Read the model definition and answer for the solid it produces. Units are mm, in the model's axes. A direction names the side the tool comes from. Give positions to 0.01 mm unless a question says otherwise; leave off trailing zeros. Loops run counter-clockwise (first coordinate to the right, second up) from the corner with the lowest first, then second, coordinate; pieces in that order, holes last. Notation, with made-up numbers: M 84,7.5 L 134,7.5 A28 cw 134,44.5 Z; hole C 69,86 d6. An arc over 180 degrees is marked long. Return JSON: item names as keys, results as strings. Group by question number.
```python
from build123d import *

# Parameters (mm, degrees)
F0_R     = 17.5
F1_DEPTH = 75
F4_R     = 15
F5_DEPTH = 25


with BuildPart() as f1:
    # F0 (on Top) → F1 (new body)
    with BuildSketch(Plane.XY):
        Circle(F0_R)
    extrude(amount=F1_DEPTH)

    # F2 (on Front) → F3 (revolve)
    with BuildSketch(Plane.XZ):
        Polygon((-19.5, 74), (0, 74), (0, 123), (-16.75, 123), (-23.75, 116), (-23.75, 104), (-19.5, 99.75), align=None)
    revolve(axis=Axis((0, 0, 40.698601), (0, 0, 1)))

    # F4 (on face) → F5 (join)
    with BuildSketch(Plane.XY.offset(123)):
        Circle(F4_R)
    extrude(amount=F5_DEPTH)


solid = f1.part
```
1. Straight lines are drawn through the part: line 1 along Z through (x, y) = (-3.5, 16); line 2 along Y through (x, z) = (0.5, 142); line 3 along Y through (x, z) = (0, 47). For each, find the intervals that lie inside material, in ascending order.
2. Flat-ended cylindrical pins translate along their axes: P1, Ø8, axis at x = -18.5, y = 19, coming from the -Z side; P2, Ø2, axis at x = 14.5, y = -11, coming from the +Z side; P3, Ø2, axis at y = -9, z = 28, coming from the -X side. Find the tip coordinate at first contact, or state that the pin passes through.
3. Find section A-A (y = 0). Write down the section's boundary in (x, z), and give its area (3 significant figures).
4. Find section C-C (z = 98). Write down the section's boundary in (x, y).
5. For faces 1 (the cylindrical face through (-13.887, -10.648, 36.482)), 2 (the flat face through (0, 0, 148)), 3 (the cylindrical face through (-14.985, 0.66, 135.325)), determine the directions among +Z, -Z, +X, -X, +Y, -Y from which every point of the face is accessible in a straight line to the end or side of a thin tool.
6. Find section D-D (z = 59). Write down the section's boundary in (x, y).
Result:
{
 "1": {"line 1": "z = 0 to 123", "line 2": "y = -14.99 to 14.99", "line 3": "y = -17.5 to 17.5"},
 "2": {"P1": "stops at z = 102.77", "P2": "stops at z = 122.55", "P3": "stops at x = -15.56"},
 "3": {"outline": "M -23.75,104 L -19.5,99.75 L -19.5,74 L -17.5,74 L -17.5,0 L 17.5,0 L 17.5,74 L 19.5,74 L 19.5,99.75 L 23.75,104 L 23.75,116 L 16.75,123 L 15,123 L 15,148 L -15,148 L -15,123 L -16.75,123 L -23.75,116 Z", "area": "5,380 mm2"},
 "4": {"outline": "C 0,0 d39"},
 "5": {"face 1": "-Z", "face 2": "+Z, +X, -X, +Y, -Y", "face 3": "+Z"},
 "6": {"outline": "C 0,0 d35"}
}
